```python
from build123d import *

# Parameters (mm, degrees)
SKETCH_R          = 0.75
PAD_DEPTH         = 1
SKETCH001_R       = 1.5
PAD001_DEPTH      = 2
PAD002_DEPTH      = 2
SKETCH003_R       = 0.45
PAD003_DEPTH      = 3
PAD003_DEPTH_BACK = 3.75
FILLET_R          = 0.4


with BuildPart() as part:
    # Sketch → Pad (new body)
    with BuildSketch(Plane.XY):
        with BuildLine():
            ThreePointArc((10.84, -2.1), (12.94, 0), (10.84, 2.1))
            Line((10.84, 2.1), (-10.84, 2.1))
            ThreePointArc((-10.84, 2.1), (-12.94, 0), (-10.84, -2.1))
            Line((10.84, -2.1), (-10.84, -2.1))
        make_face()
        with Locations((-11.49, 0)):
            Circle(SKETCH_R, mode=Mode.SUBTRACT)
        with Locations((11.49, 0)):
            Circle(SKETCH_R, mode=Mode.SUBTRACT)
    extrude(amount=-PAD_DEPTH)

    # Sketch001 → Pad001 (join)
    with BuildSketch(Plane.XY):
        with BuildLine():
            ThreePointArc((-7.94, 2.1), (-10.04, 0), (-7.94, -2.1))
            Line((-7.94, -2.1), (7.94, -2.1))
            ThreePointArc((7.94, -2.1), (10.04, 0), (7.94, 2.1))
            Line((-7.94, 2.1), (7.94, 2.1))
        make_face()
        with Locations((-7.94, 0)):
            Circle(SKETCH001_R, mode=Mode.SUBTRACT)
        with Locations((7.94, 0)):
            Circle(SKETCH001_R, mode=Mode.SUBTRACT)
    extrude(amount=PAD001_DEPTH)

    # Sketch002 → Pad002 (join)
    with BuildSketch(Plane.XY):
        with BuildLine():
            ThreePointArc((-7.939999, 2.1), (-10.039999, 0), (-7.939999, -2.1))
            Line((-7.939999, -2.1), (7.94, -2.1))
            ThreePointArc((7.94, -2.1), (10.04, 0), (7.94, 2.1))
            Line((-7.939999, 2.1), (7.94, 2.1))
        make_face()
    extrude(amount=-PAD002_DEPTH)

    # Sketch003 → Pad003 (join, two sides)
    with BuildSketch(Plane.XY) as pad003_sk:
        with Locations((-5.08, 0)):
            Circle(SKETCH003_R)
        with Locations((-2.54, 0)):
            Circle(SKETCH003_R)
        Circle(SKETCH003_R)
        with Locations((2.54, 0)):
            Circle(SKETCH003_R)
        with Locations((5.08, 0)):
            Circle(SKETCH003_R)
    extrude(amount=PAD003_DEPTH)
    extrude(pad003_sk.sketch, amount=-PAD003_DEPTH_BACK)

    # Fillet
    fillet_edges = [part.edges().sort_by_distance(p)[0] for p in [
        (-5.53, 0, 3),
        (-2.99, 0, 3),
        (-0.45, 0, 3),
        (2.09, 0, 3),
        (4.63, 0, 3),
    ]]
    fillet(fillet_edges, radius=FILLET_R)


solid = part.part
```
Part model, mm, in its own coordinate system. A direction names the side the tool comes from. Coordinates: 2 decimals unless noted, no trailing zeros. Write each loop counter-clockwise with the first axis right and the second up, starting at its lowest first coordinate (ties: lowest second). Pieces come first, ordered by that corner, then holes.
Item 1: Slice it at A-A (z = -2.25). Write the cut outline in (x, y), and give its area (3 significant figures).
Item 2: Slice it at D-D (y = 1.8). Write the cut outline in (x, z).
Item 3: Which spindle directions (+Z, -Z, +X, -X, +Y, -Y) get a long thin tool onto all of the face, cutting with end or side? Do faces 1 (the face through (0, -1, -2)), 2 (the face through (2.5, 0, -3.75)), 3 (the face through (-2.99, 0.02, 2.3)), 4 (the face through (10.04, -0.05, -1.49)). Say none if no direction does.
Item 4: Slice it at B-B (z = -0.75). Write the cut outline in (x, y), and give its area (3 significant figures).
Item 5: Slice it at C-C (x = 11.49). Write the cut outline in (y, z), and give its area (3 significant figures).
Item 6: Pin check, flat tips, straight feed: pin 1 (2 mm diameter, centred on y = -1, z = -0.5, fed in from -X); pin 2 (1.3 mm diameter, centred on x = 4.5, y = -1, fed in from -Z); pin 3 (1.4 mm diameter, centred on x = 11.49, y = 0, fed in from +Z); pin 4 (1.7 mm diameter, centred on x = -11.49, y = 0, fed in from +Z). Stop position of each tip, or through.
Item 7: Mould opens along X. For faces 5 (the face through (10.4, 0, -1)), 6 (the face through (-10.04, 0.05, 0.99)), 7 (the face through (-9.44, 0.07, 0.99)), 8 (the face through (-4.651, 0.135, 2.296)) say: released by +X, released by -X, zero draft, split by the parting line, or undercut.
Item 8: Probe line 1 (X direction, y = 0.75, z = 0.75); line 2 (X direction, y = 1.15, z = 0.25); line 3 (Y direction, x = 11.49, z = -0.55). List the from-to ranges inside material, lowest first.
Results found:
1. outline: circle Ø0.9 at (-5.08, 0); circle Ø0.9 at (-2.54, 0); circle Ø0.9 at (0, 0); circle Ø0.9 at (2.54, 0); circle Ø0.9 at (5.08, 0)
1. area: 3.18 mm2
2. outline: (-11.92, -1) - (-9.02, -1) - (-9.02, -2) - (9.02, -2) - (9.02, -1) - (11.92, -1) - (11.92, 0) - (9.02, 0) - (9.02, 2) - (-9.02, 2) - (-9.02, 0) - (-11.92, 0) - close
3. face 1: -Z
3. face 2: -Z, +X, -X, +Y, -Y
3. face 3: +Z
3. face 4: -Z, +X
4. outline: (-10.84, -2.1) - (10.84, -2.1) arc R2.1 ccw to (10.84, 2.1) - (-10.84, 2.1) arc R2.1 ccw to start; hole circle Ø1.5 at (-11.49, 0); hole circle Ø1.5 at (11.49, 0)
4. area: 101 mm2
5. outline: (-2, -1) - (-0.75, -1) - (-0.75, 0) - (-2, 0) - close; (0.75, -1) - (2, -1) - (2, 0) - (0.75, 0) - close
5. area: 2.49 mm2
6. pin 1: stops at x = -12.94
6. pin 2: stops at z = -2
6. pin 3: passes through
6. pin 4: stops at z = 0
7. face 5: zero draft
7. face 6: released by -X
7. face 7: undercut
7. face 8: undercut
8. line 1: x = -9.9 to -9.24, -6.64 to 6.64, 9.24 to 9.9
8. line 2: x = -9.7 to -8.9, -6.98 to 6.98, 8.9 to 9.7
8. line 3: y = -2 to -0.75, 0.75 to 2
